Can you work these out from the model? Positions are in its coordinate system, mm. Face numbers are marked on the shaded views. A direction names the side the tool comes from. Give positions to 0.01 mm unless a question says otherwise; leave off trailing zeros. Loops run counter-clockwise (first coordinate to the right, second up) from the corner with the lowest first, then second, coordinate; pieces in that order, holes last. Notation, with made-up numbers: M 16.25,61 L 64.25,61 A15 ccw 64.25,70 Z; hole C -31.75,-2 d3. An arc over 180 degrees is marked long. Put each result on its own line as item: value. Start each with the question number.
1) Please list where these lines run through material, in increasing order: line 1 along Z through (x, y) = (0, -14.5); line 2 along Z through (x, y) = (0.5, -4.5); line 3 along Y through (x, z) = (2, 14). Write a range as from..to.
2) Imagine slicing it at C-C (z = 38.5). Write out the boundary of the cut face in (x, y).
3) For the marked faces 4, 5, 6 and 7, which set-ups out of +Z, -Z, +X, -X, +Y, -Y let a thin tool reach every point of the face, with its end or its side?
4) If we mould it in two halves opening along X, with no side actions, what happens to the marked faces 1, 2 and 3? For each: +X half, -X half, draft (parallel to the pull), parting line (faces both ways), or undercut.
5) Imagine slicing it at B-B (x = 0). Write out the boundary of the cut face in (y, z), then the cut area to 3 significant figures.
6) For P1, Ø20, axis at x = 9, z = 37, coming from the -Y side; P2, Ø1.5, axis at x = 20, z = 65, coming from the -Y side; P3, Ø12, axis at x = -17, y = -14.5, coming from the +Z side, each with a flat end and sliding along its axis, tell me the tip position at first contact or that it passes through.
7) Imagine slicing it at D-D (y = -32). Write out the boundary of the cut face in (x, z).
from build123d import *

# Parameters (mm, degrees)
F0_R     = 20
F0_R_2   = 10
F1_DEPTH = 28
F2_DEPTH = 12
F3_DEPTH = 40


# Not quite as in the source:
# - ends of sketch curves that miss each other by under 0.0002 mm in the source are joined


with BuildPart() as f1:
    # F0 (on Front) → F1 (new body)
    with BuildSketch(Plane.XZ):
        with Locations((0, 36.7759418548)):
            Circle(F0_R)
        with Locations((0, 36.7759418548)):
            Circle(F0_R_2, mode=Mode.SUBTRACT)
    extrude(amount=F1_DEPTH)

    # F0 (on Front) → F2 (join)
    with BuildSketch(Plane.XZ):
        with BuildLine():
            ThreePointArc((40, 36.7759418548), (0, 76.7759418548), (-40, 36.7759418548))
            Line((-40, 36.7759418548), (-40.0000252162, -3.2240581452))
            Line((-40.0000252162, -3.2240581452), (39.9999747838, -3.2240581452))
            Line((39.9999747838, -3.2240581452), (40, 36.7759418548))
        make_face()
        with Locations((0, 36.7759418548)):
            Circle(F0_R, mode=Mode.SUBTRACT)
    extrude(amount=F2_DEPTH)

    # F0 (on Front) → F3 (join)
    with BuildSketch(Plane.XZ):
        Polygon((39.9999747838, -3.2240581452), (-40, -3.2240581452), (-40.0000441283, -33.2240581452), (-20.0000441283, -33.2240707533), (-20.0000346722, -18.2240707533), (19.9999653278, -18.2240623479), (19.9999558717, -33.2240623479), (39.9999558717, -33.2240581452), align=None)
    extrude(amount=F3_DEPTH)


solid = f1.part
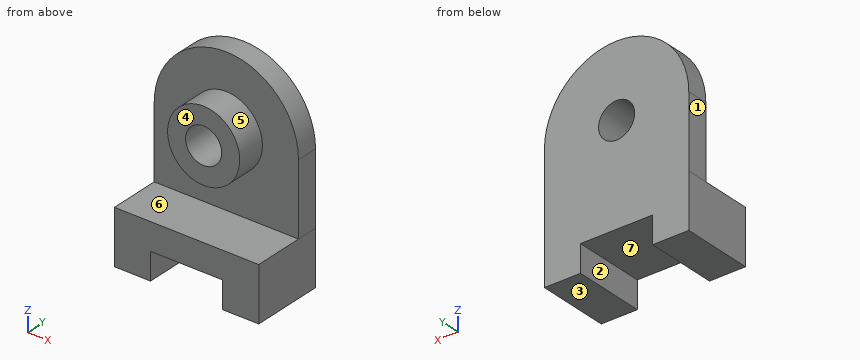
Recorded:
1. line 1: -18.22..-3.22, 16.78..26.78, 46.78..56.78
1. line 2: -18.22..26.79, 46.76..76.77
1. line 3: -12..0
2. outline: M -39.96,-12 L -19.93,-12 L -19.93,-28 L -9.85,-28 L -9.85,0 L -39.96,0 Z; M 9.85,-28 L 19.93,-28 L 19.93,-12 L 39.96,-12 L 39.96,0 L 9.85,0 Z
3. face 4: +Z, +X, -X, -Y
3. face 5: -Y
3. face 6: +X, -X, -Y
3. face 7: -Z, +Y, -Y
4. face 1: -X half
4. face 2: undercut
4. face 3: draft
5. outline: M -40,-18.22 L 0,-18.22 L 0,26.78 L -28,26.78 L -28,16.78 L -12,16.78 L -12,-3.22 L -40,-3.22 Z; M -28,46.78 L 0,46.78 L 0,76.78 L -12,76.78 L -12,56.78 L -28,56.78 Z
5. area: 1,640 mm²
6. P1: y = -28
6. P2: y = -12
6. P3: z = 75.07
7. outline: M -40,-33.22 L -20,-33.22 L -20,-18.22 L 20,-18.22 L 20,-33.22 L 40,-33.22 L 40,-3.22 L -40,-3.22 Z
